Verification items for the finished model (mm, model axes). A direction names the side the tool comes from. Round coordinates to 2 decimals unless told otherwise and drop trailing zeros. Order: outer loops, then holes, each group sorted by start corner. A loop starts at its lowest first (then second) coordinate and runs counter-clockwise, first axis right, second up. Notation, with made-up numbers: M 82.5,19.25 L 109.5,19.25 A31 cw 109.5,47.25 Z; hole C 34.5,13 d7. An arc over 180 degrees is marked long. One line per item, written item: value. Start each with the question number.
from build123d import *

# Parameters (mm, degrees)
SKETCH_1_W          = 20
SKETCH_1_H          = 20
SKETCH_1_W_2        = 16
SKETCH_1_H_2        = 16
EXTRUDE_1_DEPTH     = 275
SKETCH_4_R          = 2.5
CUT_EXTRUDE_3_DEPTH = 84
SKETCH_5_R          = 2.5
CUT_EXTRUDE_4_DEPTH = 276.907593226
SKETCH_6_R          = 2.5
CUT_EXTRUDE_5_DEPTH = 20


with BuildPart() as part:
    # 草图1 → 凸台-拉伸1 (new body)
    with BuildSketch(Plane.XY):
        Rectangle(SKETCH_1_W, SKETCH_1_H)
        Rectangle(SKETCH_1_W_2, SKETCH_1_H_2, mode=Mode.SUBTRACT)
    extrude(amount=EXTRUDE_1_DEPTH)

    # 草图4 → 切除-拉伸3 (cut)
    with BuildSketch(Plane.ZY.offset(10)):
        with Locations(Location((107.5, 0, 0), (0, 0, 270))):
            Circle(SKETCH_4_R)
        with Locations(Location((167.5, 0, 0), (0, 0, 270))):
            Circle(SKETCH_4_R)
        with Locations(Location((137.5, 0, 0), (0, 0, 270))):
            Circle(SKETCH_4_R)
    extrude(amount=-CUT_EXTRUDE_3_DEPTH, mode=Mode.SUBTRACT)

    # 草图5 → 切除-拉伸4 (cut, through all)
    with BuildSketch(Plane(origin=(10, 0, 0), x_dir=(0, 0, -1), z_dir=(1, 0, 0))):
        with Locations((-77.5, 0)):
            Circle(SKETCH_5_R)
        with Locations((-57.5, 0)):
            Circle(SKETCH_5_R)
        with Locations((-37.5, 0)):
            Circle(SKETCH_5_R)
        with Locations(Location((-237.5, 0, 0), (0, 0, 90))):
            Circle(SKETCH_5_R)
        with Locations(Location((-217.5, 0, 0), (0, 0, 90))):
            Circle(SKETCH_5_R)
        with Locations(Location((-197.5, 0, 0), (0, 0, 90))):
            Circle(SKETCH_5_R)
    extrude(amount=-CUT_EXTRUDE_4_DEPTH, mode=Mode.SUBTRACT)

    # 草图6 → 切除-拉伸5 (cut)
    with BuildSketch(Plane(origin=(0, 10, 0), x_dir=(1, 0, 0), z_dir=(0, 1, 0))):
        with Locations(Location((0, -267.5, 0), (0, 0, 270))):
            Circle(SKETCH_6_R)
        with Locations(Location((0, -252.5, 0), (0, 0, 270))):
            Circle(SKETCH_6_R)
        with Locations(Location((0, -22.5, 0), (0, 0, 270))):
            Circle(SKETCH_6_R)
        with Locations(Location((0, -7.5, 0), (0, 0, 270))):
            Circle(SKETCH_6_R)
    extrude(amount=-CUT_EXTRUDE_5_DEPTH, mode=Mode.SUBTRACT)


solid = part.part
1. Scan lines: line 1 along X through (y, z) = (5.5, 110); line 2 along X through (y, z) = (-8.7, 7.5). Record each from-to range of solid material in increasing order.
2. Tool access check on faces 4 (the face through (0, -8, 136)), 5 (the face through (-9, 0, 0)). Record the directions out of +Z, -Z, +X, -X, +Y, -Y that give a thin tool (end or side, any length) a straight path to the whole face; none if there is none.
3. Draft check along X on faces 1 (the face through (10, -2.4, 135.6)), 2 (the face through (0.751, 9.014, 9.885)), 3 (the face through (-9, 0, 140)). Enter one of: released by +X, released by -X, zero draft, split by the parting line, or undercut.
4. Section check C-C (z = 258). Record the cut outline in (x, y), and give its area (3 significant figures).
5. Section check B-B (y = 5.5). Record the cut outline in (x, z).
6. Section check D-D (x = 0). Give the number of separate pieces and of enclosed holes in the cut face, and give its area (3 significant figures).
7. Section check A-A (z = 22.5). Record the cut outline in (x, y).
Geometry check:
1. line 1: x = -10 to -8, 8 to 10
1. line 2: x = -10 to -2.5, 2.5 to 10
2. face 4: +Z, -Z
2. face 5: -Z, +X, -X, +Y, -Y
3. face 1: released by +X
3. face 2: undercut
3. face 3: zero draft
4. outline: M -10,-10 L 10,-10 L 10,10 L -10,10 Z; hole M -8,-8 L 8,-8 L 8,8 L -8,8 Z
4. area: 144 mm²
5. outline: M -10,0 L -8,0 L -8,275 L -10,275 Z; M 8,0 L 10,0 L 10,275 L 8,275 Z
6. separate pieces: 10
6. enclosed holes: 0
6. area: 1,020 mm²
7. outline: M -10,-10 L -2.5,-10 L -2.5,-8 L -8,-8 L -8,8 L -2.5,8 L -2.5,10 L -10,10 Z; M 2.5,-10 L 10,-10 L 10,10 L 2.5,10 L 2.5,8 L 8,8 L 8,-8 L 2.5,-8 Z
